The listing builds one solid part. Answer for the finished solid, in the listing's coordinates (mm). Face numbers are marked on the shaded views. Coordinates: 2 decimals unless noted, no trailing zeros. Order: outer loops, then holes, each group sorted by start corner. A loop starts at its lowest first (then second) coordinate and runs counter-clockwise, first axis right, second up. Notation, with made-up numbers: (60, 75) -> (75, 75) arc R25 ccw to (75, 106) -> close; hole circle Ø7 at (84, -32.5). An arc over 180 degrees is marked (long way). Answer in a Markdown table with one row per item.
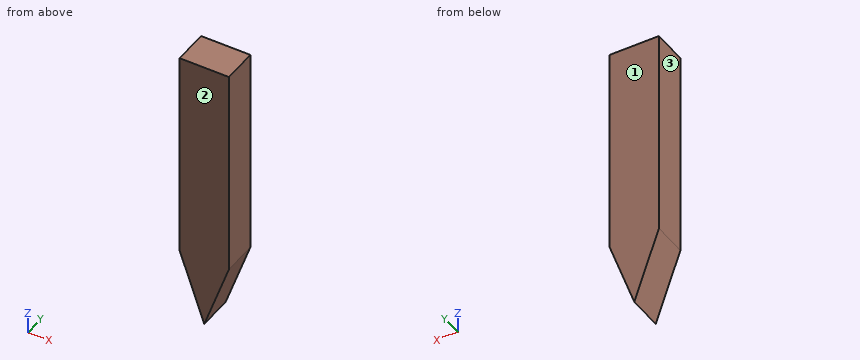
```python
from build123d import *

# Parameters (mm, degrees)
F0_W     = 88.9
F0_H     = 38.1000016469
F1_DEPTH = 508
F3_DEPTH = 25.4
F4_DEPTH = 38.1010016469


with BuildPart() as f1:
    # F0 (on Top) → F1 (new body)
    with BuildSketch(Plane.XY):
        with Locations((-261.9274258614, -47.6780477911)):
            Rectangle(F0_W, F0_H)
    extrude(amount=F1_DEPTH)

    # F2 (on face) → F3 (join)
    with BuildSketch(Plane.XZ.offset(66.7280486146)):
        Polygon((-306.3774258614, 508), (-306.3774258614, 127), (-261.9274258614, 0), (-217.4774258614, 127), (-217.4774258614, 508), align=None)
    extrude(amount=F3_DEPTH)

    # F4 (cut, through all): faces of the model
    f4_faces = [f1.faces().sort_by_distance(p)[0] for p in [
        (-291.5607591947, -66.7280486146, 42.3333333333),
        (-232.294092528, -66.7280486146, 42.3333333333),
    ]]
    extrude(f4_faces, amount=-F4_DEPTH, mode=Mode.SUBTRACT)


solid = f1.part
```
(1) Find the intervals of material crossed by line 1 along X through (y, z) = (-32.5, 114); line 2 along X through (y, z) = (-33, 113.5), in increasing order. Write a range as from..to.
Check values:
| item | result |
|---|---|
| line 1 | -301.83..-222.03 |
| line 2 | -301.65..-222.2 |
(2) A cutting plane is placed at C-C, the plane z = 104.5. Determine the outline of the cut face in (x, y).
Check values:
| item | result |
|---|---|
| outline | (-298.5, -92.13) -> (-225.35, -92.13) -> (-225.35, -28.63) -> (-298.5, -28.63) -> close |
(3) For a pull along Y with two mould halves and no side action, classify the marked faces 1, 2 and 3 as released by +Y, released by -Y, zero draft, split by the parting line, or undercut.
Check values:
| item | result |
|---|---|
| face 1 | released by +Y |
| face 2 | released by -Y |
| face 3 | zero draft |
(4) A cutting plane is placed at B-B, the plane x = -245. Determine the outline of the cut face in (y, z), then the cut area to 3 significant figures.
Check values:
| item | result |
|---|---|
| outline | (-92.13, 48.36) -> (-28.63, 48.36) -> (-28.63, 508) -> (-92.13, 508) -> close |
| area | 29,200 mm² |
(5) A cutting plane is placed at A-A, the plane y = -49. Determine the outline of the cut face in (x, z).
Check values:
| item | result |
|---|---|
| outline | (-306.38, 127) -> (-261.93, 0) -> (-217.48, 127) -> (-217.48, 508) -> (-306.38, 508) -> close |
